Check sheet for the modelled part. Datum: model origin and axes. Units: mm. Face numbers are marked on the shaded views. A direction names the side the tool comes from. Round coordinates to 2 decimals unless told otherwise and drop trailing zeros. Put each result on its own line as item: value. Start each with the question number.
```python
from build123d import *

# Parameters (mm, degrees)
SKETCH_1_R          = 1.55
EXTRUDE_1_DEPTH     = 20
SKETCH_3_R          = 1.55
EXTRUDE_2_DEPTH     = 25
FILLET_1_R          = 2
CUT_EXTRUDE_1_DEPTH = 15
CUT_EXTRUDE_START   = 15.4
CUT_EXTRUDE_2_DEPTH = 15.4


with BuildPart() as part:
    # 草图1 → 凸台-拉伸1 (new body)
    with BuildSketch(Plane.XY):
        with BuildLine():
            Line((-106.251840892, 28.470094961), (-82.103695235, 21.999618834))
            ThreePointArc((-82.103695235, 21.999618834), (-51.744721466, 67.435033925), (0, 85))
            Line((0, 85), (5, 85))
            Line((5, 85), (5, 110))
            Line((5, 110), (0, 110))
            ThreePointArc((0, 110), (-66.963757191, 87.268867432), (-106.251840892, 28.470094961))
        make_face()
        with Locations((-48.75, 84.437476869)):
            Circle(SKETCH_1_R, mode=Mode.SUBTRACT)
        with Locations((-84.437476869, 48.75)):
            Circle(SKETCH_1_R, mode=Mode.SUBTRACT)
    extrude(amount=EXTRUDE_1_DEPTH)

    # 草图3 → 凸台-拉伸2 (add)
    with BuildSketch(Plane.XZ.offset(-85)):
        with BuildLine():
            Line((43.97114317, -22.5), (61.291651246, -12.5))
            ThreePointArc((61.291651246, -12.5), (37.5, 11.291651246), (5, 20))
            Line((5, 20), (5, 0))
            ThreePointArc((5, 0), (27.5, -6.02885683), (43.97114317, -22.5))
        make_face()
        with Locations(Location((10.011455208, 12.28119514, 0), (0, 0, 270))):
            Circle(SKETCH_3_R, mode=Mode.SUBTRACT)
        with Locations(Location((45.658639918, -4.341360082, 0), (0, 0, 270))):
            Circle(SKETCH_3_R, mode=Mode.SUBTRACT)
    extrude(amount=-EXTRUDE_2_DEPTH)

    # 圆角1
    fillet_1_edges = [part.edges().sort_by_distance(p)[0] for p in [
        (-82.103695235, 21.999618834, 10),
        (-106.251840892, 28.470094961, 10),
        (43.97114317, 97.5, -22.5),
        (27.5, 85, -6.02885683),
        (52.631397208, 85, -17.5),
        (52.631397208, 110, -17.5),
        (27.5, 110, -6.02885683),
        (2.5, 110, 0),
        (2.5, 85, 0),
        (-51.744721466, 67.435033925, 0),
        (-94.177768063, 25.234856897, 0),
        (-66.963757191, 87.268867432, 0),
    ]]
    fillet(fillet_1_edges, radius=FILLET_1_R)

    # 草图4 → 切除-拉伸1 (cut)
    with BuildSketch(Plane.XY.offset(20)):
        with BuildLine():
            Line((-101.615396926, 27.227763545), (-86.740139201, 23.24195025))
            ThreePointArc((-86.740139201, 23.24195025), (-54.666776325, 71.243129958), (0, 89.8))
            Line((0, 89.8), (5, 89.8))
            Line((5, 89.8), (5, 105.2))
            Line((5, 105.2), (0, 105.2))
            ThreePointArc((0, 105.2), (-64.041702332, 83.460771399), (-101.615396926, 27.227763545))
        make_face()
    extrude(amount=-CUT_EXTRUDE_1_DEPTH, mode=Mode.SUBTRACT)

    # 草图5 → 切除-拉伸2 (cut)
    with BuildSketch(Plane.XZ.offset(-105.2).offset(CUT_EXTRUDE_START)):
        with BuildLine():
            Line((5, 20), (5, 5))
            ThreePointArc((5, 5), (30, -1.698729811), (48.301270189, -20))
            Line((48.301270189, -20), (61.291651246, -12.5))
            ThreePointArc((61.291651246, -12.5), (37.5, 11.291651246), (5, 20))
        make_face()
    extrude(amount=-CUT_EXTRUDE_2_DEPTH, mode=Mode.SUBTRACT)


solid = part.part
```
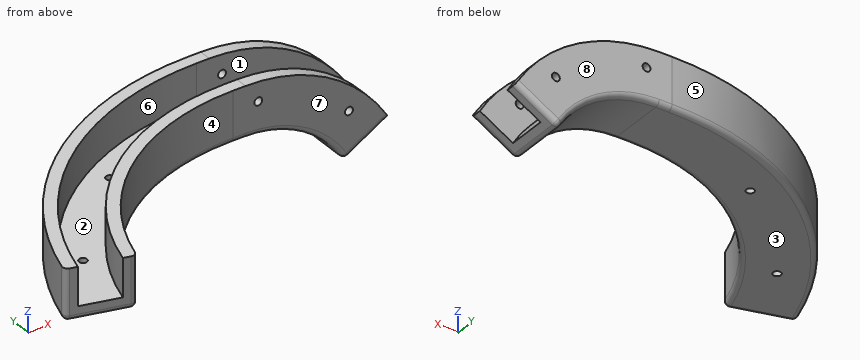
Q1. Set-up check for the marked faces 1, 2, 3, 4 and 5: record each of +Z, -Z, +X, -X, +Y, -Y from which the full face is reachable in a straight line by a thin tool's end or side.
Q2. Material ranges on line 1 (Y direction, x = 52, z = -15); line 2 (Z direction, x = -83, y = 59); line 3 (Y direction, x = -64, z = 15.5), recorded low to high. Write a range as from..to.
Q3. Draft check along Y on the marked faces 6, 7 and 8. Enter one of: +Y half, -Y half, draft (parallel to the pull), parting line (faces both ways), or undercut.
Q4. Depth check by flat-ended pin: pin 1 Ø1.9 at (x, y) = (-84.44, 48.75) entering from -Z; pin 2 Ø1 at (y, z) = (50, 3) entering from +X; pin 3 Ø4 at (x, z) = (45.66, -4.34) entering from -Y; pin 4 Ø10 at (y, z) = (93.5, -14) entering from -X. Enter the tip coordinate at first touch or a pass-through.
Answer list:
1. face 1: +Z, +X
1. face 2: +Z
1. face 3: -Z, -X, +Y, -Y
1. face 4: +Z, -Z, +X, -Y
1. face 5: +Z, -Z, -X, +Y
2. line 1: y = 85..89.8, 105.2..110
2. line 2: z = 0..5
2. line 3: y = 55.94..62.99, 83.49..89.47
3. face 6: undercut
3. face 7: -Y half
3. face 8: +Y half
4. pin 1: passes through
4. pin 2: stops at x = -68.37
4. pin 3: stops at y = 85
4. pin 4: stops at x = 32
